from build123d import *

# Parameters (mm, degrees)
F0_W     = 3.175
F0_H     = 3.175
F0_W_2   = 8.255
F0_H_2   = 15.875
F1_DEPTH = 1.5875
F0_W_3   = 3.81
F0_H_3   = 5.715
F2_DEPTH = 3.175
F0_W_4   = 19.05
F3_DEPTH = 1.5875
F4_DEPTH = 11.1125


with BuildPart() as f1:
    # F0 (on Top) → F1 (new body)
    with BuildSketch(Plane.XY):
        with Locations((-11.1125, -7.9375)):
            Rectangle(F0_W, F0_H)
        Polygon((-12.7, -6.35), (-9.525, -6.35), (-9.525, 1.5875), (-9.525, 6.35), (-9.525, 9.525), (-12.7, 9.525), align=None)
        Polygon((9.525, -6.35), (9.525, 9.525), (3.81, 9.525), (3.81, 5.715), (3.81, 0), (0, 0), (0, 5.715), (-1.27, 5.715), (-1.27, 1.5875), (-9.525, 1.5875), (-9.525, -6.35), align=None)
        with Locations((-5.3975, 7.9375)):
            Rectangle(F0_W_2, F0_H)
        Polygon((3.81, 5.715), (3.81, 9.525), (-1.27, 9.525), (-1.27, 6.35), (-1.27, 5.715), (0, 5.715), align=None)
        with Locations((11.1125, 1.5875)):
            Rectangle(F0_W, F0_H_2)
        with Locations((11.1125, -7.9375)):
            Rectangle(F0_W, F0_H)
    extrude(amount=F1_DEPTH)

    # F0 (on Top) → F2 (join)
    with BuildSketch(Plane.XY):
        Polygon((-1.27, 5.715), (-1.27, 6.35), (-9.525, 6.35), (-9.525, 1.5875), (-1.27, 1.5875), align=None)
        with Locations((1.905, 2.8575)):
            Rectangle(F0_W_3, F0_H_3)
    extrude(amount=F2_DEPTH)

    # F0 (on Top) → F3 (join)
    with BuildSketch(Plane.XY):
        with Locations((0, -7.9375)):
            Rectangle(F0_W_4, F0_H)
    extrude(amount=F3_DEPTH)

    # F0 (on Top) → F4 (join)
    with BuildSketch(Plane.XY):
        with Locations((0, -7.9375)):
            Rectangle(F0_W_4, F0_H)
    extrude(amount=-F4_DEPTH)


solid = f1.part
Check sheet for the modelled part. Datum: model origin and axes. Units: mm. A direction names the side the tool comes from. Give positions to 0.01 mm unless a question says otherwise; leave off trailing zeros. Loops run counter-clockwise (first coordinate to the right, second up) from the corner with the lowest first, then second, coordinate; pieces in that order, holes last. Notation, with made-up numbers: M 9,54.5 L 26,54.5 A20 cw 26,61.5 Z; hole C 32,38.25 d9. An arc over 180 degrees is marked long. Answer as a JSON object with one key per item and string values. Group by question number.
Q1. Cross-section at B-B on y = 2.25. Record the cut outline in (x, z) (1 decimal), then the cut area to 3 significant figures.
Q2. Material ranges on line 1 along Z through (x, y) = (4.75, 3.25); line 2 along Z through (x, y) = (7.5, -7); line 3 along Y through (x, z) = (6.25, -5) (3 decimals), recorded low to high. Write a range as [from, to].
Q3. Cross-section at D-D on y = -8. Record the cut outline in (x, z) (1 decimal).
Q4. Release check for a two-part mould opening along X. For faces 5 (the flat face through (12.7, 0, 1)), 6 (the flat face through (0, -6.35, -5)), 7 (the flat face through (-1.27, 4, 2)) record: released by +X, released by -X, zero draft, split by the parting line, or undercut.
Q5. Go/stop test with flat-tipped pins: P1, Ø4, axis at x = 4, z = -7, coming from the +Y side; P2, Ø3.5, axis at y = -8, z = -6.5, coming from the -X side (3 decimals); P3, Ø1.6, axis at y = -8.5, z = -5.5, coming from the +X side (3 decimals). Record where each tip stops, or that it passes through.
Q6. Cross-section at C-C on z = -9.5. Record the cut outline in (x, y) (3 decimals), then the cut area to 3 significant figures.
Q7. Access from +Z, -Z, +X, -X, +Y, -Y to the whole of each face (thin tool, end or side, straight path). Record for faces 1 (the flat face through (-9.525, 4, 2)), 2 (the flat face through (2, 0, 2)), 3 (the flat face through (9.525, -8, -5)), 4 (the flat face through (2, 5.715, 2)).
Evaluation:
{
 "1": {"outline": "M -12.7,0 L 12.7,0 L 12.7,1.6 L 3.8,1.6 L 3.8,3.2 L 0,3.2 L 0,1.6 L -1.3,1.6 L -1.3,3.2 L -9.5,3.2 L -9.5,1.6 L -12.7,1.6 Z", "area": "59.5 mm2"},
 "2": {"line 1": "z = [0, 1.59]", "line 2": "z = [-11.11, 1.59]", "line 3": "y = [-9.525, -6.35]"},
 "3": {"outline": "M -12.7,0 L -9.5,0 L -9.5,-11.1 L 9.5,-11.1 L 9.5,0 L 12.7,0 L 12.7,1.6 L -12.7,1.6 Z"},
 "4": {"face 5": "released by +X", "face 6": "zero draft", "face 7": "undercut"},
 "5": {"P1": "stops at y = -6.35", "P2": "stops at x = -9.525", "P3": "stops at x = 9.525"},
 "6": {"outline": "M -9.525,-9.525 L 9.525,-9.525 L 9.525,-6.35 L -9.525,-6.35 Z", "area": "60.5 mm2"},
 "7": {"face 1": "+Z, -X, +Y, -Y", "face 2": "+Z, +X, -X, -Y", "face 3": "-Z, +X, +Y, -Y", "face 4": "+Z, +X, +Y"}
}
